Geometry: final body of the model. Coordinates: model frame, mm. Round coordinates to 2 decimals unless told otherwise and drop trailing zeros. Write each loop counter-clockwise with the first axis right and the second up, starting at its lowest first coordinate (ties: lowest second). Pieces come first, ordered by that corner, then holes. Notation, with made-up numbers: (71, 82.25) -> (88, 82.25) arc R19 ccw to (88, 94.25) -> close; hole circle Ø2 at (78.25, 62.5). An arc over 180 degrees is marked (long way). Use one line per item in the form item = value. Start each with the question number.
1. Line query: L1, parallel to Z at x = -40, y = 2; L2, parallel to X at y = 1.5, z = -69; L3, parallel to Z at x = 0, y = 2.75. Output: solid intervals per line, ascending.
2. Draft query along X for faces 1 (the face through (-2, 3, -74)), 2 (the face through (110, 3, 1)), 3 (the face through (-58.973, 1.75, 67.141)). Return one class per face: pulls with the +X half, pulls with the -X half, needs draft (parallel to the pull), parting line crosses it, or undercut.
3. Cut plane B-B, the plane y = 5. State how many separate pieces and enclosed holes the cut face has, plus the area to 3 significant figures.
4. Cut plane A-A, the plane z = 69. Return the cut outline in (x, y), plus the area to 3 significant figures.
5. Pin query (flat end, axial travel): pin 1 Ø9 at (x, z) = (-61, 69) entering from -Y; pin 2 Ø4.5 at (x, z) = (103, 69) entering from -Y; pin 3 Ø7 at (x, z) = (-101, 69) entering from +Y. Return the tip coordinate at first contact, or that it passes through.
```python
from build123d import *

# Parameters (mm, degrees)
SKETCH1_W                                       = 220
SKETCH1_H                                       = 148
BOSS_EXTRUDE1_DEPTH                             = 6
CSK_FOR_M5_FLAT_HEAD_MACHINE_SCREW2_D           = 5.5
CSK_FOR_M5_FLAT_HEAD_MACHINE_SCREW2_CSINK_D     = 10.4
CSK_FOR_M5_FLAT_HEAD_MACHINE_SCREW2_CSINK_ANGLE = 90
F_4_0MM_DOWEL_HOLE1_D                           = 4
F_4_0MM_DOWEL_HOLE1_DEPTH                       = 12
F_4_0MM_DOWEL_HOLE1_TIP                         = 1.201721238
F_4_0MM_DOWEL_HOLE2_AT_2_COUNT                  = 2
F_4_0MM_DOWEL_HOLE2_AT_2_PITCH                  = 23
F_4_0MM_DOWEL_HOLE2_AT_3_COUNT                  = 2
F_4_0MM_DOWEL_HOLE2_AT_3_PITCH                  = 33
F_4_0MM_DOWEL_HOLE2_AT_4_COUNT                  = 2
F_4_0MM_DOWEL_HOLE2_AT_4_PITCH                  = 34.481879299
F_4_0MM_DOWEL_HOLE2_AT_5_COUNT                  = 2
F_4_0MM_DOWEL_HOLE2_AT_5_PITCH                  = 59.908263203
F_4_0MM_DOWEL_HOLE2_AT_6_COUNT                  = 2
F_4_0MM_DOWEL_HOLE2_AT_6_PITCH                  = 89
F_4_0MM_DOWEL_HOLE2_AT_7_COUNT                  = 2
F_4_0MM_DOWEL_HOLE2_AT_7_PITCH                  = 66


with BuildPart() as part:
    # Sketch1 → Boss-Extrude1 (new body)
    with BuildSketch(Plane(origin=(0, 0, 0), x_dir=(1, 0, 0), z_dir=(0, 1, 0))):
        Rectangle(SKETCH1_W, SKETCH1_H)
    extrude(amount=BOSS_EXTRUDE1_DEPTH)

    # CSK for M5 Flat Head Machine Screw2 (through all)
    with Locations(Plane(origin=(0, 6, 0), x_dir=(1, 0, 0), z_dir=(0, 1, 0))):
        with Locations((103, -69), (63, -69), (-101, -69), (-61, -69), (103, 69), (63, 69), (-61, 69), (-101, 69)):
            CounterSinkHole(CSK_FOR_M5_FLAT_HEAD_MACHINE_SCREW2_D / 2, CSK_FOR_M5_FLAT_HEAD_MACHINE_SCREW2_CSINK_D / 2, counter_sink_angle=CSK_FOR_M5_FLAT_HEAD_MACHINE_SCREW2_CSINK_ANGLE)

    # Ø4.0mm Dowel Hole1
    with Locations(Plane(origin=(0, 6, 0), x_dir=(1, 0, 0), z_dir=(0, 1, 0))):
        with Locations((0, 56), (0, 33), (0, -33), (0, -56)):
            Hole(F_4_0MM_DOWEL_HOLE1_D / 2, depth=F_4_0MM_DOWEL_HOLE1_DEPTH)
            with Locations((0, 0, -(F_4_0MM_DOWEL_HOLE1_DEPTH + F_4_0MM_DOWEL_HOLE1_TIP / 2))):  # 118° drill point
                Cone(0, F_4_0MM_DOWEL_HOLE1_D / 2, F_4_0MM_DOWEL_HOLE1_TIP, mode=Mode.SUBTRACT)

    # Sketch8 → Ø4.0mm Dowel Hole2 (revolve, cut)
    with BuildSketch(Plane(origin=(-40, 6, -33), x_dir=(0, 0, 1), z_dir=(1, 0, 0))):
        Polygon((0, 0), (0, 13.201721238), (2, 12), (2, 0), align=None)
    f_4_0mm_dowel_hole2 = revolve(axis=Axis((-40, 12.35, -33), (0, -1, 0)), mode=Mode.SUBTRACT)

    # Ø4.0mm Dowel Hole2 at 2: Ø4.0mm Dowel Hole2 ×2
    with Locations(*[(0, 0, -i * F_4_0MM_DOWEL_HOLE2_AT_2_PITCH) for i in range(1, F_4_0MM_DOWEL_HOLE2_AT_2_COUNT)]):
        add(f_4_0mm_dowel_hole2, mode=Mode.SUBTRACT)

    # Ø4.0mm Dowel Hole2 at 3: Ø4.0mm Dowel Hole2 ×2
    with Locations(*[(0, 0, i * F_4_0MM_DOWEL_HOLE2_AT_3_PITCH) for i in range(1, F_4_0MM_DOWEL_HOLE2_AT_3_COUNT)]):
        add(f_4_0mm_dowel_hole2, mode=Mode.SUBTRACT)

    # Ø4.0mm Dowel Hole2 at 4: Ø4.0mm Dowel Hole2 ×2
    with Locations(*[Vector(-0.290007395, 0, 0.957024404) * (i * F_4_0MM_DOWEL_HOLE2_AT_4_PITCH) for i in range(1, F_4_0MM_DOWEL_HOLE2_AT_4_COUNT)]):
        add(f_4_0mm_dowel_hole2, mode=Mode.SUBTRACT)

    # Ø4.0mm Dowel Hole2 at 5: Ø4.0mm Dowel Hole2 ×2
    with Locations(*[Vector(-0.834609407, 0, 0.550842208) * (i * F_4_0MM_DOWEL_HOLE2_AT_5_PITCH) for i in range(1, F_4_0MM_DOWEL_HOLE2_AT_5_COUNT)]):
        add(f_4_0mm_dowel_hole2, mode=Mode.SUBTRACT)

    # Ø4.0mm Dowel Hole2 at 6: Ø4.0mm Dowel Hole2 ×2
    with Locations(*[(0, 0, i * F_4_0MM_DOWEL_HOLE2_AT_6_PITCH) for i in range(1, F_4_0MM_DOWEL_HOLE2_AT_6_COUNT)]):
        add(f_4_0mm_dowel_hole2, mode=Mode.SUBTRACT)

    # Ø4.0mm Dowel Hole2 at 7: Ø4.0mm Dowel Hole2 ×2
    with Locations(*[(0, 0, i * F_4_0MM_DOWEL_HOLE2_AT_7_PITCH) for i in range(1, F_4_0MM_DOWEL_HOLE2_AT_7_COUNT)]):
        add(f_4_0mm_dowel_hole2, mode=Mode.SUBTRACT)

    # Mirror1: Ø4.0mm Dowel Hole2 across plane
    add(f_4_0mm_dowel_hole2.mirror(Plane(origin=(0, 0, 0), x_dir=(0, 0, 1), z_dir=(1, 0, 0))), mode=Mode.SUBTRACT)

    # Mirror1 copy 1 sketch → Mirror1 copy 1 (revolve, cut)
    with BuildSketch(Plane(origin=(40, 6, -56), x_dir=(0, 0, 1), z_dir=(-1, 0, 0))):
        Polygon((0, 0), (0, -13.201721238), (2, -12), (2, 0), align=None)
    revolve(axis=Axis((40, 12.35, -56), (0, 1, 0)), mode=Mode.SUBTRACT)

    # Mirror1 copy 2 sketch → Mirror1 copy 2 (revolve, cut)
    with BuildSketch(Plane(origin=(40, 6, 0), x_dir=(0, 0, 1), z_dir=(-1, 0, 0))):
        Polygon((0, 0), (0, -13.201721238), (2, -12), (2, 0), align=None)
    revolve(axis=Axis((40, 12.35, 0), (0, 1, 0)), mode=Mode.SUBTRACT)

    # Mirror1 copy 3 sketch → Mirror1 copy 3 (revolve, cut)
    with BuildSketch(Plane(origin=(50, 6, 0), x_dir=(0, 0, 1), z_dir=(-1, 0, 0))):
        Polygon((0, 0), (0, -13.201721238), (2, -12), (2, 0), align=None)
    revolve(axis=Axis((50, 12.35, 0), (0, 1, 0)), mode=Mode.SUBTRACT)

    # Mirror1 copy 4 sketch → Mirror1 copy 4 (revolve, cut)
    with BuildSketch(Plane(origin=(90, 6, 0), x_dir=(0, 0, 1), z_dir=(-1, 0, 0))):
        Polygon((0, 0), (0, -13.201721238), (2, -12), (2, 0), align=None)
    revolve(axis=Axis((90, 12.35, 0), (0, 1, 0)), mode=Mode.SUBTRACT)

    # Mirror1 copy 5 sketch → Mirror1 copy 5 (revolve, cut)
    with BuildSketch(Plane(origin=(40, 6, 56), x_dir=(0, 0, 1), z_dir=(-1, 0, 0))):
        Polygon((0, 0), (0, -13.201721238), (2, -12), (2, 0), align=None)
    revolve(axis=Axis((40, 12.35, 56), (0, 1, 0)), mode=Mode.SUBTRACT)

    # Mirror1 copy 6 sketch → Mirror1 copy 6 (revolve, cut)
    with BuildSketch(Plane(origin=(40, 6, 33), x_dir=(0, 0, 1), z_dir=(-1, 0, 0))):
        Polygon((0, 0), (0, -13.201721238), (2, -12), (2, 0), align=None)
    revolve(axis=Axis((40, 12.35, 33), (0, 1, 0)), mode=Mode.SUBTRACT)


solid = part.part
```
Outcome:
q1.L1 = -74 to -58, -54 to -35, -31 to -2, 2 to 31, 35 to 54, 58 to 74
q1.L2 = -110 to -103.75, -98.25 to -63.75, -58.25 to 60.25, 65.75 to 100.25, 105.75 to 110
q1.L3 = -74 to -58, -54 to -35, -31 to 31, 35 to 54, 58 to 74
q2.face_1 = needs draft
q2.face_2 = pulls with the +X half
q2.face_3 = undercut
q3.separate_pieces = 1
q3.enclosed_holes = 26
q3.area = 31,900 mm^2
q4.outline = (-110, 0) -> (-103.75, 0) -> (-103.75, 3.55) -> (-106.2, 6) -> (-110, 6) -> close; (-98.25, 0) -> (-63.75, 0) -> (-63.75, 3.55) -> (-66.2, 6) -> (-95.8, 6) -> (-98.25, 3.55) -> close; (-58.25, 0) -> (60.25, 0) -> (60.25, 3.55) -> (57.8, 6) -> (-55.8, 6) -> (-58.25, 3.55) -> close; (65.75, 0) -> (100.25, 0) -> (100.25, 3.55) -> (97.8, 6) -> (68.2, 6) -> (65.75, 3.55) -> close; (105.75, 0) -> (110, 0) -> (110, 6) -> (108.2, 6) -> (105.75, 3.55) -> close
q4.area = 1,160 mm^2
q5.pin_1 = 0
q5.pin_2 = through
q5.pin_3 = 4.3
